Input: part model. Units: mm. Frame: model coordinates. Face numbers are marked on the shaded views. A direction names the side the tool comes from. Give positions to 0.01 mm unless a question says otherwise; leave off trailing zeros. Write each loop counter-clockwise with the first axis right and the second up, starting at its lowest first coordinate (ties: lowest second). Pieces come first, ordered by that corner, then holes. Notation, with made-up numbers: (82.25, -27.5) - (131.25, -27.5) arc R9 cw to (131.25, -18.5) - close; hole circle Ø10 at (41.25, 28.25). An arc over 180 degrees is marked (long way). Answer as CSV lines item,"result".
```python
from build123d import *

# Parameters (mm, degrees)
F0_W     = 101.6
F0_H     = 101.6
F2_DEPTH = 25.4
F3_DEPTH = 54.864
F4_W     = 81.382974
F4_H     = 19.05
F5_DEPTH = 25.654


with BuildPart() as f2:
    # F0 (on Top) → F2 (new body)
    with BuildSketch(Plane.XY):
        Rectangle(F0_W, F0_H)
        with BuildLine():
            ThreePointArc((50.8, -50.8), (101.6, 0), (50.8, 50.8))
            Line((50.8, 50.8), (50.8, -50.8))
        make_face()
    extrude(amount=F2_DEPTH)

    # F1 (on face) → F3 (cut)
    with BuildSketch(Plane.XY):
        with BuildLine():
            ThreePointArc((50.8, -28.476143), (62.53461, -16.334626), (66.812163, 0))
            ThreePointArc((66.812163, 0), (62.53461, 16.334626), (50.8, 28.476143))
            Line((50.8, 28.476143), (50.8, -28.476143))
        make_face()
        with BuildLine():
            Line((50.8, -28.476143), (50.8, 28.476143))
            ThreePointArc((50.8, 28.476143), (0.157828, 0), (50.8, -28.476143))
        make_face()
    extrude(amount=F3_DEPTH, mode=Mode.SUBTRACT)

    # F4 (on face) → F5 (join)
    with BuildSketch(Plane(origin=(-50.8, 0, 0), x_dir=(0, -1, 0), z_dir=(-1, 0, 0))):
        with Locations((10.108513, 53.975)):
            Rectangle(F4_W, F4_H)
        Polygon((-30.582974, 44.45), (-50.8, 44.45), (-50.8, 25.4), (50.8, 25.4), (50.8, 44.45), align=None)
    extrude(amount=-F5_DEPTH)


solid = f2.part
```
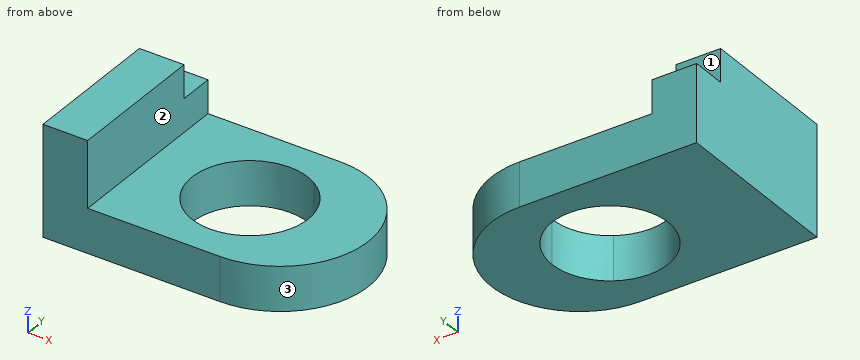
Item 1: Reachability of the marked faces 1, 2 and 3 from +Z, -Z, +X, -X, +Y, -Y: full face, straight path, thin tool, end or side. Return the list, or none.
The answers:
face 1,"+Z, +X, -X, +Y"
face 2,"+Z, +X, +Y, -Y"
face 3,"+Z, -Z, +X"
Item 2: Ray query, line 1 (Y direction, x = 33, z = 12); line 2 (Z direction, x = 13, y = 43); line 3 (X direction, y = 24.5, z = 40). Return the intervals inside material, ascending. Write a range as from..to.
The answers:
line 1,"-50.8..-33.32, 33.32..50.8"
line 2,"0..25.4"
line 3,"-50.8..-25.15"
Item 3: Contact query for flat-ended pins moving along their axis: pin 1 (3 mm diameter, centred on x = -7, y = 40.5, fed in from +Z); pin 2 (10 mm diameter, centred on x = -35.5, y = 45.5, fed in from +Z); pin 3 (21 mm diameter, centred on x = -38, z = 58, fed in from +Y). Output: stop coordinate, or through.
The answers:
pin 1,"z = 25.4"
pin 2,"z = 44.45"
pin 3,"y = 30.58"
Item 4: Cut plane D-D on z = 40.5. Return the cut outline in (x, y).
The answers:
outline,"(-50.8, -50.8) - (-25.15, -50.8) - (-25.15, 50.8) - (-50.8, 50.8) - close"
Item 5: Cut plane A-A on z = 19.5. Return the cut outline in (x, y) (3 decimals), plus the area to 3 significant figures.
The answers:
outline,"(-50.8, -50.8) - (50.8, -50.8) arc R50.8 ccw to (50.8, 50.8) - (-50.8, 50.8) - close; hole (50.8, -28.476) arc R33.327 ccw to (66.812, 0) arc R33.327 ccw to (50.8, 28.476) arc R33.327 ccw (long way) to start"
area,"10,900 mm²"
Item 6: Cut plane B-B on x = 26. Return the cut outline in (y, z).
The answers:
outline,"(-50.8, 0) - (-32.48, 0) - (-32.48, 25.4) - (-50.8, 25.4) - close; (32.48, 0) - (50.8, 0) - (50.8, 25.4) - (32.48, 25.4) - close"
Item 7: Cut plane C-C on y = -24. Return the cut outline in (x, z).
The answers:
outline,"(-50.8, 0) - (10.36, 0) - (10.36, 25.4) - (-25.15, 25.4) - (-25.15, 63.5) - (-50.8, 63.5) - close; (56.61, 0) - (95.57, 0) - (95.57, 25.4) - (56.61, 25.4) - close"
